```python
from build123d import *

# Parameters (mm, degrees)
SKETCH1_R           = 2.5
BOSS_EXTRUDE1_DEPTH = 10
CHAMFER1_SIZE       = 2
SKETCH2_R           = 6
CUT_EXTRUDE1_DEPTH  = 48
SKETCH3_R           = 6
CUT_EXTRUDE2_DEPTH  = 14
SKETCH4_R           = 2.528531427
SKETCH4_R_2         = 2.5
CUT_EXTRUDE3_DEPTH  = 14
CHAMFER2_SIZE       = 2
FILLET1_R           = 82


with BuildPart() as part:
    # Sketch1 → Boss-Extrude1 (new body)
    with BuildSketch(Plane.XY):
        with BuildLine():
            Line((55.484867262, -31.782339645), (74.83591229, -21.271406043))
            ThreePointArc((74.83591229, -21.271406043), (79.305955572, -8.361988007), (66.856482862, -2.7366))
            Line((66.856482862, -2.7366), (-123.999650399, -2.7366))
            ThreePointArc((-123.999650399, -2.7366), (-131.077427076, -5.672247424), (-133.999632379, -12.755584536))
            ThreePointArc((-133.999632379, -12.755584536), (-126.357727013, -67.682340192), (-104.205340418, -118.521488224))
            Line((-104.205340418, -118.521488224), (-30.34426595, -78.402267355))
            ThreePointArc((-30.34426595, -78.402267355), (-21.450076132, -71.83180545), (-14.694704232, -63.077233349))
            ThreePointArc((-14.694704232, -63.077233349), (5.93460242, -42.875720255), (34.110442904, -36.567674809))
            ThreePointArc((34.110442904, -36.567674809), (45.131584541, -35.666553732), (55.484867262, -31.782339645))
        make_face()
        with Locations((-122, -7.7366)):
            Circle(SKETCH1_R, mode=Mode.SUBTRACT)
        with Locations((-82, -7.7366)):
            Circle(SKETCH1_R, mode=Mode.SUBTRACT)
        with Locations((-42, -7.7366)):
            Circle(SKETCH1_R, mode=Mode.SUBTRACT)
        with Locations((-2, -7.7366)):
            Circle(SKETCH1_R, mode=Mode.SUBTRACT)
        with Locations((38, -7.7366)):
            Circle(SKETCH1_R, mode=Mode.SUBTRACT)
    extrude(amount=BOSS_EXTRUDE1_DEPTH)

    # Chamfer1
    chamfer1_edges = [part.edges().sort_by_distance(p)[0] for p in [
        (-124.5, -7.7366, 10),
        (-84.5, -7.7366, 10),
        (-44.5, -7.7366, 10),
        (-4.5, -7.7366, 10),
        (35.5, -7.7366, 10),
    ]]
    chamfer(chamfer1_edges, length=CHAMFER1_SIZE)

    # Sketch2 → Cut-Extrude1 (cut)
    with BuildSketch(Plane.XY.offset(10)):
        with Locations((70, -12.3683)):
            Circle(SKETCH2_R)
    extrude(amount=-CUT_EXTRUDE1_DEPTH, mode=Mode.SUBTRACT)

    # Sketch3 → Cut-Extrude2 (cut)
    with BuildSketch(Plane.XY.offset(10)):
        with Locations((-60, -38)):
            Circle(SKETCH3_R)
    extrude(amount=-CUT_EXTRUDE2_DEPTH, mode=Mode.SUBTRACT)

    # Sketch4 → Cut-Extrude3 (cut)
    with BuildSketch(Plane.XY.offset(10)):
        with Locations((-128.565543545, -25.510785173)):
            Circle(SKETCH4_R)
        with Locations((-124.80403691, -53.01786585)):
            Circle(SKETCH4_R_2)
        with Locations((-117.250891281, -79.733748965)):
            Circle(SKETCH4_R_2)
        with Locations((-106.053120049, -105.138440244)):
            Circle(SKETCH4_R_2)
    extrude(amount=-CUT_EXTRUDE3_DEPTH, mode=Mode.SUBTRACT)

    # Chamfer2
    chamfer2_edges = [part.edges().sort_by_distance(p)[0] for p in [
        (-131.094074972, -25.510785173, 10),
        (-127.30403691, -53.01786585, 10),
        (-119.750891281, -79.733748965, 10),
        (-108.553120049, -105.138440244, 10),
    ]]
    chamfer(chamfer2_edges, length=CHAMFER2_SIZE)

    # Fillet1
    fillet1_edges = [part.edges().sort_by_distance(p)[0] for p in [
        (66.856482862, -2.7366, 5),
    ]]
    fillet(fillet1_edges, radius=FILLET1_R)


solid = part.part
```
The model under review builds one solid part; all positions refer to its coordinate system, in mm. Give positions to 0.01 mm unless a question says otherwise; leave off trailing zeros. Write each loop counter-clockwise with the first axis right and the second up, starting at its lowest first coordinate (ties: lowest second). Pieces come first, ordered by that corner, then holes. Notation, with made-up numbers: M -32,73 L 1,73 A36 ccw 1,109 Z; hole C -29,-36.75 d2. An arc over 180 degrees is marked long. Write item = value, one per line. Start each with the question number.
Q1. Clearance check with flat-ended pins moving along their axes: pin 1 (1.5 mm diameter, centred on x = -19, z = 3.5, fed in from +Y); pin 2 (6 mm diameter, centred on x = 38, y = -7.74, fed in from +Z); pin 3 (8 mm diameter, centred on x = -2, y = -7.74, fed in from +Z); pin 4 (6 mm diameter, centred on x = -42, y = -7.74, fed in from -Z). State where each tip first meets the part, or that it passes through.
Q2. For line 1 (Y direction, x = -82, z = 5.25); line 2 (X direction, y = -41, z = 5); line 3 (Y direction, x = -55.5, z = 1), list the stretches that pass through material, from the lowest coordinate up.
Q3. We need section B-B (z = 4.5). Give the number of separate pieces and of enclosed holes in the cut face, plus the area to 3 significant figures.
Q4. We need section C-C (x = -82). State the section outline as (y, z) points, plus the area to 3 significant figures.
Q5. Mouldability with a two-part tool opening along Y and no side actions: class faces 1 (the face through (5.58, -43.07, 4.93)), 2 (the face through (-52, -47, 0)), 3 (the face through (-119.496, -6.948, 8.125)) as released by +Y, released by -Y, zero draft, split by the parting line, or undercut.
Q6. We need section D-D (x = 47). State the section outline as (y, z) points, plus the area to 3 significant figures.
Q7. We need section A-A (x = -42). State the section outline as (y, z) points, plus the area to 3 significant figures.
Result set:
q1.pin_1 = -2.74
q1.pin_2 = 8.5
q1.pin_3 = 9.5
q1.pin_4 = 0
q2.line_1 = -106.46 to -10.24, -5.24 to -2.74
q2.line_2 = -131.98 to -65.2, -54.8 to 9.75
q2.line_3 = -92.07 to -41.97, -34.03 to -2.74
q3.separate_pieces = 1
q3.enclosed_holes = 11
q3.area = 13,400 mm2
q4.outline = M -106.46,0 L -10.24,0 L -10.24,8 L -12.24,10 L -106.46,10 Z; M -5.24,0 L -2.74,0 L -2.74,10 L -3.24,10 L -5.24,8 Z
q4.area = 983 mm2
q5.face_1 = released by -Y
q5.face_2 = zero draft
q5.face_3 = undercut
q6.outline = M -35.2,0 L -2.74,0 L -2.74,10 L -35.2,10 Z
q6.area = 325 mm2
q7.outline = M -84.73,0 L -10.24,0 L -10.24,8 L -12.24,10 L -84.73,10 Z; M -5.24,0 L -2.74,0 L -2.74,10 L -3.24,10 L -5.24,8 Z
q7.area = 766 mm2
